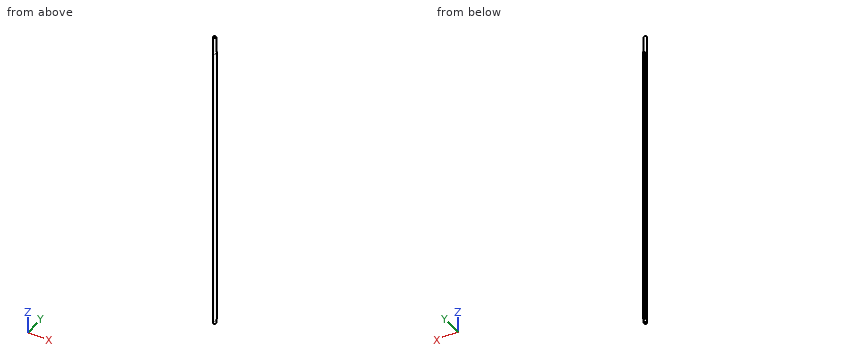
Autodesk Inventor part; units mm, degrees
ref_plane "YZ Plane" through (0, 0, 0) normal (1, 0, 0) x (0, 1, 0)
ref_plane "XZ Plane" through (0, 0, 0) normal (0, 1, 0) x (-1, 0, 0)
ref_plane "XY Plane" through (0, 0, 0) normal (0, 0, 1) x (1, 0, 0)
sketch "Sketch1" plane through (0, 0, 0) normal (0, 0, 1) x (1, 0, 0)
  arc A0 (-1, 2.2913) -> (1, 2.2913) centre (0, 0) ccw
  line L0 (-1, 5.5) -> (1, 5.5)
  line L1 (1, 5.5) -> (1, 2.2913)
  line L2 (-1, 2.2913) -> (-1, 5.5)
  line L3 (-1, 5.5) -> (1, 2.5) construction
  line L4 (1, 5.5) -> (-1, 2.5) construction
  point P0 (0, 4)
  dimension "d0" = 5
extrude "Extrusion1" add sketch "Sketch1" against normal blind 494
sketch "Sketch2" plane through (0, 0, 0) normal (0, 0, 1) x (1, 0, 0)
  circle A0 centre (0, 0) radius 2.5
  dimension "d3" = 5
extrude "Extrusion2" add sketch "Sketch2" along normal blind 30
sketch "Sketch3" plane through (0, 0, -494) normal (0, 0, -1) x (-1, 0, 0)
  circle A0 centre (0, 0) radius 2.5
  dimension "d6" = 5
extrude "Extrusion3" add sketch "Sketch3" along normal blind 5
properties part number "shaft"
Design review of the part built by this model. Coordinates are the model's own, in mm. Give positions to 0.01 mm unless a question says otherwise; leave off trailing zeros. Write each loop counter-clockwise with the first axis right and the second up, starting at its lowest first coordinate (ties: lowest second). Pieces come first, ordered by that corner, then holes.
(1) Add section A-A (x = 0). Give the boundary of the cut face in (y, z).
Checked values:
outline: (-2.5, -499) - (2.5, -499) - (2.5, -494) - (5.5, -494) - (5.5, 0) - (2.5, 0) - (2.5, 30) - (-2.5, 30) - close
(2) Clearance check with flat-ended pins moving along their axes: pin 1 Ø3 at (x, z) = (1.5, -248) entering from +Y; pin 2 Ø0.6 at (x, y) = (-0.5, 4.5) entering from +Z; pin 3 Ø2.5 at (y, z) = (4, -175.5) entering from +X; pin 4 Ø1.6 at (y, z) = (3.5, -144) entering from -X. State where each tip first meets the part, or that it passes through.
Checked values:
pin 1: stops at y = 5.5
pin 2: stops at z = 0
pin 3: stops at x = 1
pin 4: stops at x = -1
(3) Add section B-B (z = -338.5). Give the boundary of the cut face in (x, y), and give its area (3 significant figures).
Checked values:
outline: (-1, 2.29) arc R2.5 ccw (long way) to (1, 2.29) - (1, 5.5) - (-1, 5.5) - close
area: 25.8 mm2
(4) Wall thickness on line 1 along Y through (x, z) = (-2.25, -474.5); line 2 along Y through (x, z) = (0.1, -160); line 3 along X through (y, z) = (0.25, -185): over which ranges is each line inside the solid? List them lowest first.
Checked values:
line 1: y = -1.09 to 1.09
line 2: y = -2.5 to 5.5
line 3: x = -2.49 to 2.49
